```python
from build123d import *

# Parameters (mm, degrees)
CYLINDER016_R     = 1.5
CYLINDER016_DEPTH = 20
CYLINDER017_R     = 1.5
CYLINDER017_DEPTH = 20
BOX006_W          = 30
BOX006_H          = 34
BOX006_DEPTH      = 1.5


with BuildPart() as cylinder016:
    # Cylinder016 → Cylinder016 (new body)
    with BuildSketch(Plane(origin=(2, 15.25, 20), x_dir=(1, 0, 0), z_dir=(0, 0, 1))):
        Circle(CYLINDER016_R)
    extrude(amount=CYLINDER016_DEPTH)


with BuildPart() as fusion004:
    # Cylinder017 → Cylinder017 (new body)
    with BuildSketch(Plane(origin=(20, 15.25, 20), x_dir=(1, 0, 0), z_dir=(0, 0, 1))):
        Circle(CYLINDER017_R)
    extrude(amount=CYLINDER017_DEPTH)

    # Fusion004: union Cylinder016
    add(cylinder016.part)


with BuildPart() as sup_gps_b:
    # Box006 → Box006 (new body)
    with BuildSketch(Plane(origin=(-1.5, 12, 35), x_dir=(1, 0, 0), z_dir=(0, 0, 1))):
        with Locations((15, 17)):
            Rectangle(BOX006_W, BOX006_H)
    extrude(amount=BOX006_DEPTH)

    # Cut004: cut Fusion004
    add(fusion004.part, mode=Mode.SUBTRACT)


solid = sup_gps_b.part
```
Geometry: final body of the model. Coordinates: model frame, mm. Coordinates: 2 decimals unless noted, no trailing zeros. Loops run counter-clockwise (first coordinate to the right, second up) from the corner with the lowest first, then second, coordinate; pieces in that order, holes last. Notation, with made-up numbers: M 3,-15 L 33,-15 A26 cw 33,23 Z; hole C -4,11 d4. An arc over 180 degrees is marked long. Put each result on its own line as item: value.
(1) Cut plane B-B on y = 15.25. Return the cut outline in (x, z).
Answer sheet:
outline: M -1.5,35 L 0.5,35 L 0.5,36.5 L -1.5,36.5 Z; M 3.5,35 L 18.5,35 L 18.5,36.5 L 3.5,36.5 Z; M 21.5,35 L 28.5,35 L 28.5,36.5 L 21.5,36.5 Z
(2) Material intervals for probe 1 along X at (y, z) = (15.25, 36.05); probe 2 along Y at (x, z) = (2, 36.05), sorted ascending.
Answer sheet:
probe 1: x = -1.5 to 0.5, 3.5 to 18.5, 21.5 to 28.5
probe 2: y = 12 to 13.75, 16.75 to 46
(3) Draft query along X for faces 1 (the face through (0.89, 16.26, 35.74)), 2 (the face through (-1.5, 29, 36)), 3 (the face through (28.5, 29, 36)). Return one class per face: pulls with the +X half, pulls with the -X half, needs draft (parallel to the pull), parting line crosses it, or undercut.
Answer sheet:
face 1: undercut
face 2: pulls with the -X half
face 3: pulls with the +X half
(4) Cut plane A-A on x = 20. Return the cut outline in (y, z).
Answer sheet:
outline: M 12,35 L 13.75,35 L 13.75,36.5 L 12,36.5 Z; M 16.75,35 L 46,35 L 46,36.5 L 16.75,36.5 Z
